Autodesk Inventor part; units mm, degrees
ref_plane "YZ Plane" through (0, 0, 0) normal (1, 0, 0) x (0, 1, 0)
ref_plane "XZ Plane" through (0, 0, 0) normal (0, 1, 0) x (-1, 0, 0)
ref_plane "XY Plane" through (0, 0, 0) normal (0, 0, 1) x (1, 0, 0)
sketch "Sketch1" plane through (0, 0, 0) normal (0, 0, 1) x (1, 0, 0)
  line L0 (10.9384, 8.2044) -> (170.9384, 8.2044)
  line L1 (170.9384, 8.2044) -> (170.9384, 98.2044)
  line L2 (10.9384, 98.2044) -> (10.9384, 8.2044)
  line L3 (10.9384, 98.2044) -> (60.9384, 158.2044)
  line L4 (60.9384, 158.2044) -> (120.9384, 158.2044)
  line L5 (120.9384, 158.2044) -> (170.9384, 98.2044)
  dimension "d0" = 160
  dimension "d4" = 60
  dimension "d5" = 50
  dimension "d6" = 90
  dimension "d7" = 90
  dimension "d8" = 150
extrude "Extrusion1" add sketch "Sketch1" along normal blind 2.6568
sketch "Sketch2" plane through (0, 0, 2.6568) normal (0, 0, 1) x (1, 0, 0)
  line L0 (10.9384, 8.2044) -> (10.9384, 98.2044)
  line L1 (170.9384, 8.2044) -> (10.9384, 8.2044)
  circle A0 centre (20.9384, 20.9044) radius 3.57
  circle A1 centre (20.9384, 85.5044) radius 2.625
  dimension "d11" = 7.14
  dimension "d12" = 12.7
  dimension "d13" = 10
  dimension "d14" = 10
  dimension "d15" = 64.6
  dimension "d16" = 5.25
extrude "wheel_holes" cut sketch "Sketch2" against normal through all
pattern_linear "Rectangular Pattern1" count 2 spacing 140 along (1, 0, 0) of "wheel_holes"
sketch "Sketch3" plane through (0, 0, 2.6568) normal (0, 0, 1) x (1, 0, 0)
  line L0 (10.9384, 8.2044) -> (10.9384, 98.2044)
  line L1 (170.9384, 8.2044) -> (10.9384, 8.2044)
  arc A0 (79.4384, 85.5044) -> (102.4384, 85.5044) centre (90.9384, 85.5044) ccw
  arc A1 (73.8194, 100.9984) -> (77.0694, 100.9984) centre (75.4444, 100.9984) ccw
  line L2 (170.9384, 98.2044) -> (170.9384, 8.2044)
  arc A2 (77.0694, 110.9984) -> (73.8194, 110.9984) centre (75.4444, 110.9984) ccw
  line L3 (77.0694, 110.9984) -> (77.0694, 100.9984)
  line L4 (73.8194, 110.9984) -> (73.8194, 100.9984)
  arc A3 (102.4384, 95.5044) -> (79.4384, 95.5044) centre (90.9384, 95.5044) ccw
  line L5 (79.4384, 95.5044) -> (79.4384, 85.5044)
  line L6 (102.4384, 85.5044) -> (102.4384, 95.5044)
  arc A4 (104.8074, 100.9984) -> (108.0574, 100.9984) centre (106.4324, 100.9984) ccw
  arc A5 (108.0574, 110.9984) -> (104.8074, 110.9984) centre (106.4324, 110.9984) ccw
  line L7 (108.0574, 110.9984) -> (108.0574, 100.9984)
  line L8 (104.8074, 110.9984) -> (104.8074, 100.9984)
  arc A6 (73.8194, 70.0104) -> (77.0694, 70.0104) centre (75.4444, 70.0104) ccw
  arc A7 (77.0694, 80.0104) -> (73.8194, 80.0104) centre (75.4444, 80.0104) ccw
  line L9 (77.0694, 80.0104) -> (77.0694, 70.0104)
  line L10 (73.8194, 80.0104) -> (73.8194, 70.0104)
  arc A8 (104.8074, 70.0104) -> (108.0574, 70.0104) centre (106.4324, 70.0104) ccw
  arc A9 (108.0574, 80.0104) -> (104.8074, 80.0104) centre (106.4324, 80.0104) ccw
  line L11 (108.0574, 80.0104) -> (108.0574, 70.0104)
  line L12 (104.8074, 80.0104) -> (104.8074, 70.0104)
  dimension "d22" = 23
  dimension "d23" = 80
  dimension "d24" = 77.3
  dimension "d33" = 3.25
  dimension "d35" = 64.506
  dimension "d36" = 92.794
  dimension "d105" = 10
  dimension "d106" = 64.506
  dimension "d110" = 3.25
  dimension "d112" = 23
  dimension "d113" = 80
  dimension "d114" = 10
  dimension "d126" = 30.988
  dimension "d129" = 30.988
  dimension "d141" = 10
extrude "Nema_17" cut sketch "Sketch3" against normal through all
sketch "Sketch4" plane through (0, 0, 2.6568) normal (0, 0, 1) x (1, 0, 0)
  circle A0 centre (160.9384, 85.5044) radius 2.625
  circle A1 centre (20.9384, 85.5044) radius 2.625
  line L0 (10.9384, 8.2044) -> (10.9384, 98.2044)
  line L1 (170.9384, 98.2044) -> (170.9384, 8.2044)
  circle A2 centre (60.9384, 84.0044) radius 2.625
  circle A3 centre (120.9384, 84.0044) radius 2.625
  dimension "d39" = 50
  dimension "d41" = 5.25
  dimension "d42" = 50
  dimension "d43" = 1.5
  dimension "d44" = 5.25
  dimension "d99" = 1.5
extrude "Idler_Holes" cut sketch "Sketch4" against normal through all contours A2 | A3
sketch "Sketch5" plane through (0, 0, 2.6568) normal (0, 0, 1) x (1, 0, 0)
  line L0 (60.9384, 158.2044) -> (120.9384, 158.2044)
  circle A0 centre (110.9384, 148.2044) radius 2.625
  circle A1 centre (110.9384, 128.2044) radius 2.625
  circle A2 centre (70.9384, 148.2044) radius 2.625
  circle A3 centre (70.9384, 128.2044) radius 2.625
  line L1 (70.9384, 150.8294) -> (110.9384, 150.8294)
  line L2 (110.9384, 145.5794) -> (70.9384, 145.5794)
  line L3 (70.9384, 130.8294) -> (110.9384, 130.8294)
  line L4 (110.9384, 125.5794) -> (70.9384, 125.5794)
  dimension "d47" = 10
  dimension "d48" = 10
  dimension "d49" = 20
  dimension "d50" = 10
  dimension "d51" = 5.25
  dimension "d52" = 5.25
  dimension "d87" = 40
  dimension "d145" = 40
  dimension "d146" = 40
extrude "x-slot" cut sketch "Sketch5" against normal through all
fillet "Fillet2" radius 3.175 6 edges at (120.9384, 158.2044, 1.3284) (60.9384, 158.2044, 1.3284) (170.9384, 98.2044, 1.3284) (170.9384, 8.2044, 1.3284) (10.9384, 98.2044, 1.3284) (10.9384, 8.2044, 1.3284)
sketch "Sketch7" plane through (0, 0, 0) normal (0, 0, -1) x (-1, 0, 0)
  line L0 (-10.9384, 97.0549) -> (-10.9384, 11.3794)
  line L1 (-170.9384, 11.3794) -> (-170.9384, 97.0549)
  line L2 (-14.1134, 8.2044) -> (-167.7634, 8.2044)
  circle A0 centre (-140.9384, 20.9044) radius 2.625
  circle A1 centre (-40.9384, 20.9044) radius 2.625
  dimension "d68" = 5.25
  dimension "d69" = 12.7
  dimension "d70" = 30
  dimension "d71" = 5.25
  dimension "d72" = 30
  dimension "d73" = 12.7
extrude "two_plater" cut sketch "Sketch7" against normal through all
pattern_linear "Rectangular Pattern3" count 2 spacing 61.5 along (0, 1, 0) of "two_plater"
sketch "Sketch8" plane through (0, 0, 2.6568) normal (0, 0, 1) x (1, 0, 0)
  line L0 (167.7634, 8.2044) -> (14.1134, 8.2044)
  line L1 (10.9384, 11.3794) -> (10.9384, 97.0549)
  arc A0 (14.3759, 50.7044) -> (17.5009, 50.7044) centre (15.9384, 50.7044) ccw
  arc A1 (17.5009, 62.7044) -> (14.3759, 62.7044) centre (15.9384, 62.7044) ccw
  line L2 (14.3759, 50.7044) -> (14.3759, 62.7044)
  line L3 (17.5009, 62.7044) -> (17.5009, 50.7044)
  arc A2 (164.3759, 50.7044) -> (167.5009, 50.7044) centre (165.9384, 50.7044) ccw
  arc A3 (167.5009, 62.7044) -> (164.3759, 62.7044) centre (165.9384, 62.7044) ccw
  line L4 (164.3759, 50.7044) -> (164.3759, 62.7044)
  line L5 (167.5009, 62.7044) -> (167.5009, 50.7044)
  point P0 (0, 0)
  dimension "d76" = 3.125
  dimension "d77" = 3.125
  dimension "d78" = 12
  dimension "d79" = 5
  dimension "d80" = 42.5
  dimension "d81" = 3.125
  dimension "d82" = 5
  dimension "d94" = 150
extrude "limit_switches" cut sketch "Sketch8" against normal through all
sketch "Sketch10" plane through (0, 0, 2.6568) normal (0, 0, 1) x (1, 0, 0)
  line L0 (167.7634, 8.2044) -> (14.1134, 8.2044)
  line L1 (170.9384, 97.0549) -> (170.9384, 11.3794)
  arc A0 (65.9384, 20.8294) -> (65.9384, 15.5794) centre (65.9384, 18.2044) ccw
  arc A1 (115.9384, 15.5794) -> (115.9384, 20.8294) centre (115.9384, 18.2044) ccw
  line L2 (65.9384, 20.8294) -> (115.9384, 20.8294)
  line L3 (115.9384, 15.5794) -> (65.9384, 15.5794)
  point P0 (0, 0)
  dimension "d132" = 5.25
  dimension "d133" = 5.25
  dimension "d134" = 10
  dimension "d135" = 10
  dimension "d136" = 50
  dimension "d138" = 55
  dimension "d169" = 50
extrude "Extrusion10" cut sketch "Sketch10" against normal through all
sketch "Sketch11" plane through (0, 0, 2.6568) normal (0, 0, 1) x (1, 0, 0)
  line L0 (62.4255, 158.2044) -> (119.4513, 158.2044)
  line L1 (10.9384, 11.3794) -> (10.9384, 97.0549)
  circle A0 centre (60.9384, 138.2044) radius 2.625
  circle A1 centre (120.9384, 138.2044) radius 2.625
  point P0 (0, 0)
  dimension "d147" = 5.25
  dimension "d148" = 5.25
  dimension "d149" = 60
  dimension "d150" = 20
  dimension "d151" = 20
  dimension "d152" = 50
extrude "Extrusion11" cut sketch "Sketch11" against normal through all
sketch "Sketch13" plane through (0, 0, 2.6568) normal (0, 0, 1) x (1, 0, 0)
  line L0 (10.9384, 11.3794) -> (10.9384, 97.0549)
  arc A0 (102.4384, 95.5044) -> (79.4384, 95.5044) centre (90.9384, 95.5044) ccw
  arc A1 (69.9934, 118.603) -> (64.7015, 119.052) centre (67.3684, 119.0744) ccw
  arc A2 (64.7435, 114.0524) -> (69.9934, 114.0744) centre (67.3684, 114.0744) ccw
  line L1 (69.9934, 118.603) -> (69.9934, 114.0744)
  line L2 (64.7435, 114.0524) -> (64.7015, 119.052)
  point P0 (0, 0)
  dimension "d155" = 5.334
  dimension "d156" = 56.43
  dimension "d157" = 23.57
  dimension "d166" = 5.25
  dimension "d167" = 5
  dimension "d168" = 56.43
extrude "Extrusion12" cut sketch "Sketch13" against normal through all
pattern_linear "Rectangular Pattern4" count 2 spacing 47.14 along (1, 0, 0) count 2 spacing 47.14 along (0, -1, 0) of "Extrusion12"
equation "\"d7\" = d6"
equation "\"d35\" = d29"
equation "\"d112\" = d22"
equation "\"d113\" = d23"
equation "\"d42\" = d39"
equation "\"d43\" = d99"
equation "\"d44\" = d41"
equation "\"d50\" = d48"
equation "\"d52\" = d51"
equation "\"d76\" = d77"
equation "\"d82\" = d79"
equation "\"d134\" = d135"
properties part number "26029-01" material "Steel, Mild"
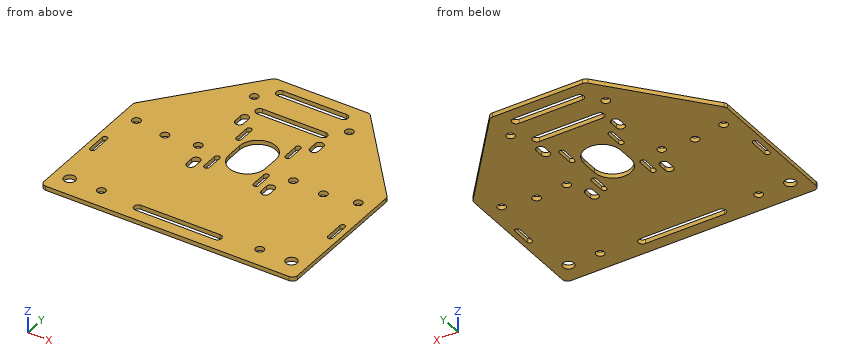
For this review, take the finished solid that the model builds, in its own axes (mm). Coordinates: 2 decimals unless noted, no trailing zeros. Loops run counter-clockwise (first coordinate to the right, second up) from the corner with the lowest first, then second, coordinate; pieces in that order, holes last.
1. Insertion check: P1, Ø7, axis at x = 160.94, y = 85.5, coming from the -Z side; P2, Ø1.3, axis at y = 107.5, z = 1.5, coming from the -X side; P3, Ø0.8, axis at y = 117, z = 1, coming from the -X side; P4, Ø1, axis at y = 113, z = 1.5, coming from the -X side. Each pin has a flat end and moves straight along its axis. Give the tip position at first contact, or say it passes through.
2. Add section A-A, the plane y = 60. Give the boundary of the cut face in (x, z).
3. Add section C-C, the plane y = 128.5. Give the boundary of the cut face in (x, z).
4. Add section B-B, the plane x = 83.5. Give the boundary of the cut face in (y, z), then the cut area to 3 significant figures.
5. Add section D-D, the plane x = 140.5. Give the boundary of the cut face in (y, z).
6. For line 1 (Y direction, x = 111, z = 1.85); line 2 (Y direction, x = 75.5, z = 0.8); line 3 (Y direction, x = 107, z = 1.9), list the stretches that pass through material, from the lowest coordinate up.
Result:
1. P1: stops at z = 0
1. P2: stops at x = 18.14
1. P3: stops at x = 26.27
1. P4: stops at x = 22.85
2. outline: (10.94, 0) - (14.38, 0) - (14.38, 2.66) - (10.94, 2.66) - close; (17.5, 0) - (164.38, 0) - (164.38, 2.66) - (17.5, 2.66) - close; (167.5, 0) - (170.94, 0) - (170.94, 2.66) - (167.5, 2.66) - close
3. outline: (36.18, 0) - (68.33, 0) - (68.33, 2.66) - (36.18, 2.66) - close; (113.55, 0) - (145.69, 0) - (145.69, 2.66) - (113.55, 2.66) - close
4. outline: (8.2, 0) - (15.58, 0) - (15.58, 2.66) - (8.2, 2.66) - close; (20.83, 0) - (76.73, 0) - (76.73, 2.66) - (20.83, 2.66) - close; (104.27, 0) - (125.58, 0) - (125.58, 2.66) - (104.27, 2.66) - close; (130.83, 0) - (145.58, 0) - (145.58, 2.66) - (130.83, 2.66) - close; (150.83, 0) - (158.2, 0) - (158.2, 2.66) - (150.83, 2.66) - close
4. area: 284 mm2
5. outline: (8.2, 0) - (18.32, 0) - (18.32, 2.66) - (8.2, 2.66) - close; (23.49, 0) - (79.82, 0) - (79.82, 2.66) - (23.49, 2.66) - close; (84.99, 0) - (134.73, 0) - (134.73, 2.66) - (84.99, 2.66) - close
6. line 1: y = 8.2 to 15.58, 20.83 to 125.58, 130.83 to 145.58, 150.83 to 158.2
6. line 2: y = 8.2 to 15.58, 20.83 to 68.39, 81.63 to 99.37, 112.62 to 125.58, 130.83 to 145.58, 150.83 to 158.2
6. line 3: y = 8.2 to 15.58, 20.83 to 68.49, 81.53 to 99.48, 112.52 to 125.58, 130.83 to 145.58, 150.83 to 158.2
